Work out the finished part from the listing and answer in its coordinate system (mm). Give positions to 0.01 mm unless a question says otherwise; leave off trailing zeros. Loops run counter-clockwise (first coordinate to the right, second up) from the corner with the lowest first, then second, coordinate; pieces in that order, holes last. Notation, with made-up numbers: M 59,16.5 L 81,16.5 A13 cw 81,23.5 Z; hole C 39,59 d8. An arc over 180 degrees is marked long. Use a Markdown table: item, result.
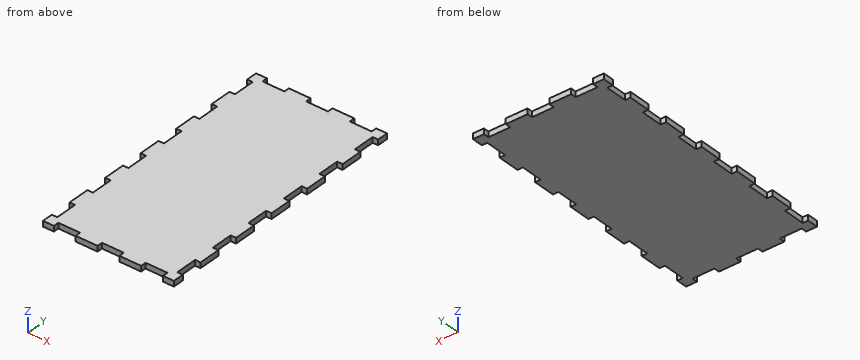
```python
from build123d import *

# Parameters (mm, degrees)
SKETCH1_W            = 76.2
SKETCH1_H            = 152.4
EXTRUDE1_DEPTH       = 3.175
SKETCH3_W            = 3.175
SKETCH3_H            = 12.7
CUT_EXTRUDE1_DEPTH   = 3.175
LPATTERN1_COUNT      = 6
LPATTERN1_PITCH      = 25.4
LPATTERN1_COUNT_DIR2 = 2
LPATTERN1_PITCH_DIR2 = 73.025
SKETCH4_W            = 12.7
SKETCH4_H            = 3.175
CUT_EXTRUDE2_DEPTH   = 3.175
LPATTERN2_COUNT      = 3
LPATTERN2_PITCH      = 25.4
LPATTERN2_COUNT_DIR2 = 2
LPATTERN2_PITCH_DIR2 = 149.225


with BuildPart() as part:
    # Sketch1 → Extrude1 (new body)
    with BuildSketch(Plane.XY):
        with Locations((38.1, 76.2)):
            Rectangle(SKETCH1_W, SKETCH1_H)
    extrude(amount=EXTRUDE1_DEPTH)

    # Sketch3 → Cut-Extrude1 (cut)
    with BuildSketch(Plane.XY.offset(3.175)):
        with Locations((74.6125, 139.7)):
            Rectangle(SKETCH3_W, SKETCH3_H)
    cut_extrude1 = extrude(amount=-CUT_EXTRUDE1_DEPTH, mode=Mode.SUBTRACT)

    # LPattern1: Cut-Extrude1 6 × 2
    with Locations(*[(-j * LPATTERN1_PITCH_DIR2, -i * LPATTERN1_PITCH, 0) for i in range(LPATTERN1_COUNT) for j in range(LPATTERN1_COUNT_DIR2) if (i, j) != (0, 0)]):
        add(cut_extrude1, mode=Mode.SUBTRACT)

    # Sketch4 → Cut-Extrude2 (cut)
    with BuildSketch(Plane.XY.offset(3.175)):
        with Locations((63.5, 150.8125)):
            Rectangle(SKETCH4_W, SKETCH4_H)
    cut_extrude2 = extrude(amount=-CUT_EXTRUDE2_DEPTH, mode=Mode.SUBTRACT)

    # LPattern2: Cut-Extrude2 3 × 2
    with Locations(*[(-i * LPATTERN2_PITCH, -j * LPATTERN2_PITCH_DIR2, 0) for i in range(LPATTERN2_COUNT) for j in range(LPATTERN2_COUNT_DIR2) if (i, j) != (0, 0)]):
        add(cut_extrude2, mode=Mode.SUBTRACT)


solid = part.part
```
(1) Given P1, Ø1.6, axis at y = 117.5, z = 1, coming from the +X side (3 decimals); P2, Ø1.6, axis at y = 142.5, z = 1.5, coming from the -X side (3 decimals), each flat-ended and moving along its own axis, determine where each tip first touches the part or whether it passes through.
Entries:
| item | result |
|---|---|
| P1 | stops at x = 73.025 |
| P2 | stops at x = 3.175 |
(2) Consider probe 1 along X at (y, z) = (95, 1.1) (3 decimals); probe 2 along Y at (x, z) = (35, 1.45) (3 decimals). Determine where each line is inside the solid, lowest interval first. Write a range as [from, to].
Entries:
| item | result |
|---|---|
| probe 1 | x = [3.175, 73.025] |
| probe 2 | y = [3.175, 149.225] |
(3) A cutting plane is placed at B-B (y = 15). Write down the section's boundary in (x, z) (3 decimals).
Entries:
| item | result |
|---|---|
| outline | M 3.175,0 L 73.025,0 L 73.025,3.175 L 3.175,3.175 Z |
(4) A cutting plane is placed at A-A (x = 59.5). Write down the section's boundary in (y, z) (3 decimals), and give its area (3 significant figures).
Entries:
| item | result |
|---|---|
| outline | M 3.175,0 L 149.225,0 L 149.225,3.175 L 3.175,3.175 Z |
| area | 464 mm² |
